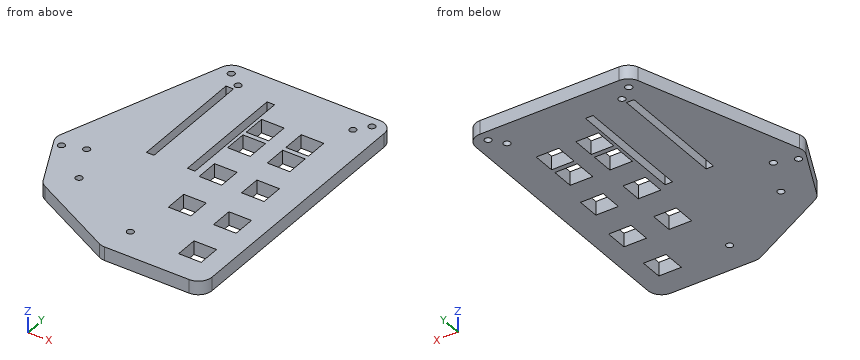
```python
from build123d import *

# Parameters (mm, degrees)
SKETCH1_R           = 1.27
BOSS_EXTRUDE1_DEPTH = 5.08
SKETCH5_W           = 8.382
SKETCH5_H           = 8.382
SKETCH5_W_2         = 2.794
SKETCH5_H_2         = 43.434
CUT_EXTRUDE1_DEPTH  = 6.08
SKETCH7_R           = 1.27
CUT_EXTRUDE3_DEPTH  = 6.08


with BuildPart() as part:
    # Sketch1 → Boss-Extrude1 (new body)
    with BuildSketch(Plane.XY):
        with BuildLine():
            Line((-3.314058103, 6.35), (48.26, 6.35))
            ThreePointArc((48.26, 6.35), (51.852102448, 4.862102448), (53.34, 1.27))
            Line((53.34, 1.27), (53.34, -92.71))
            ThreePointArc((53.34, -92.71), (51.852102448, -96.302102448), (48.26, -97.79))
            Line((48.26, -97.79), (16.846989059, -97.79))
            ThreePointArc((16.846989059, -97.79), (15.638688158, -97.644208035), (14.499741809, -97.215200367))
            Line((14.499741809, -97.215200367), (-16.7505185, -80.933552139))
            ThreePointArc((-16.7505185, -80.933552139), (-18.059258376, -79.955412607), (-18.989802686, -78.61241436))
            Line((-18.989802686, -78.61241436), (-28.309569459, -59.040904135))
            ThreePointArc((-28.309569459, -59.040904135), (-28.795802898, -57.127870198), (-28.51617555, -55.173917704))
            Line((-28.51617555, -55.173917704), (-8.107195629, 2.952923842))
            ThreePointArc((-8.107195629, 2.952923842), (-6.251501454, 5.414614163), (-3.314058103, 6.35))
        make_face()
        with Locations((48.0822, 2.286)):
            Circle(SKETCH1_R, mode=Mode.SUBTRACT)
        with Locations((-3.718687848, 1.651)):
            Circle(SKETCH1_R, mode=Mode.SUBTRACT)
        with Locations((-25.012261453, -59.761967182)):
            Circle(SKETCH1_R, mode=Mode.SUBTRACT)
    extrude(amount=BOSS_EXTRUDE1_DEPTH)

    # Sketch5 → Cut-Extrude1 (cut, through all)
    with BuildSketch(Plane(origin=(0, 0, 0), x_dir=(-1, 0, 0), z_dir=(0, 0, -1))):
        with Locations((-36.83, -17.78)):
            Rectangle(SKETCH5_W, SKETCH5_H)
        with Locations((-39.37, -45.72)):
            Rectangle(SKETCH5_W, SKETCH5_H)
        with Locations((-36.83, -27.94)):
            Rectangle(SKETCH5_W, SKETCH5_H)
        with Locations((-41.91, -64.77)):
            Rectangle(SKETCH5_W, SKETCH5_H)
        with Locations((-41.91, -83.82)):
            Rectangle(SKETCH5_W, SKETCH5_H)
        with Locations((-22.098, -17.78)):
            Rectangle(SKETCH5_W, SKETCH5_H)
        with Locations((-22.098, -27.94)):
            Rectangle(SKETCH5_W, SKETCH5_H)
        with Locations((-23.622, -45.72)):
            Rectangle(SKETCH5_W, SKETCH5_H)
        with Locations((-25.146, -64.77)):
            Rectangle(SKETCH5_W, SKETCH5_H)
        with Locations((-15.367, -26.543)):
            Rectangle(SKETCH5_W_2, SKETCH5_H_2)
        with Locations((-0.127, -26.543)):
            Rectangle(SKETCH5_W_2, SKETCH5_H_2)
    extrude(amount=-CUT_EXTRUDE1_DEPTH, mode=Mode.SUBTRACT)

    # Sketch7 → Cut-Extrude3 (cut, through all)
    with BuildSketch(Plane.XY.offset(5.08)):
        with Locations((44.2976, -2.4892)):
            Circle(SKETCH7_R)
        with Locations((1.6002, -2.4384)):
            Circle(SKETCH7_R)
        with Locations((-17.4498, -57.15)):
            Circle(SKETCH7_R)
        with Locations((-10.5918, -71.3486)):
            Circle(SKETCH7_R)
        with Locations((18.796, -86.5378)):
            Circle(SKETCH7_R)
    extrude(amount=-CUT_EXTRUDE3_DEPTH, mode=Mode.SUBTRACT)


solid = part.part
```
The model under review builds one solid part; all positions refer to its coordinate system, in mm. Round coordinates to 2 decimals unless told otherwise and drop trailing zeros. Loops run counter-clockwise (first coordinate to the right, second up) from the corner with the lowest first, then second, coordinate; pieces in that order, holes last. Notation, with made-up numbers: M -4,-11.5 L 21,-11.5 A31 ccw 21,12.5 Z; hole C 2,-37.5 d3. An arc over 180 degrees is marked long. Answer as a JSON object with one key per item and string values.
(1) Take a section at B-B on y = -57.15. Give the boundary of the cut face in (x, z).
Resolved:
{"outline": "M -28.79,0 L -18.72,0 L -18.72,5.08 L -28.79,5.08 Z; M -16.18,0 L 53.34,0 L 53.34,5.08 L -16.18,5.08 Z"}
(2) Take a section at D-D on x = -15. Give the boundary of the cut face in (y, z), and give its area (3 significant figures).
Resolved:
{"outline": "M -81.85,0 L -16.68,0 L -16.68,5.08 L -81.85,5.08 Z", "area": "331 mm²"}
(3) Take a section at A-A on x = 24.5. Give the boundary of the cut face in (y, z), and give its area (3 significant figures).
Resolved:
{"outline": "M -97.79,0 L -68.96,0 L -68.96,5.08 L -97.79,5.08 Z; M -60.58,0 L -49.91,0 L -49.91,5.08 L -60.58,5.08 Z; M -41.53,0 L -32.13,0 L -32.13,5.08 L -41.53,5.08 Z; M -23.75,0 L -21.97,0 L -21.97,5.08 L -23.75,5.08 Z; M -13.59,0 L 6.35,0 L 6.35,5.08 L -13.59,5.08 Z", "area": "359 mm²"}
(4) To check wall thickness, follow line 1 along X through (y, z) = (-20, 0.35); line 2 along Y through (x, z) = (25, 4.2); line 3 along Y through (x, z) = (36, 1.5). State the ranges of each line that lie inside material, in increasing order.
Resolved:
{"line 1": "-16.17 to -1.27, 1.52 to 13.97, 16.76 to 17.91, 26.29 to 32.64, 41.02 to 53.34", "line 2": "-97.79 to -68.96, -60.58 to -49.91, -41.53 to -32.13, -23.75 to -21.97, -13.59 to 6.35", "line 3": "-97.79 to -49.91, -41.53 to -32.13, -23.75 to -21.97, -13.59 to 6.35"}
(5) Clearance check with flat-ended pins moving along their axes: P1, Ø1.5, axis at x = -17.45, y = -57.15, coming from the -Z side; P2, Ø2.5, axis at y = -28.5, z = 1.5, coming from the -X side; P3, Ø2, axis at y = -14, z = 2, coming from the -X side; P4, Ø2, axis at y = -36.5, z = 1.5, coming from the -X side. State where each tip first meets the part, or that it passes through.
Resolved:
{"P1": "through", "P2": "x = -19.59", "P3": "x = -14.41", "P4": "x = -22.31"}
(6) Take a section at C-C on z = 2.35. Count the separate pieces of the cut face and the enclosed holes in it, and give its area (3 significant figures).
Resolved:
{"separate pieces": "1", "enclosed holes": "19", "area": "6,340 mm²"}
